```python
from build123d import *

# Parameters (mm, degrees)
SKETCH_1_R           = 11.65
SKETCH_1_R_2         = 1.8
EXTRUDE_1_DEPTH      = 170
SHELL_2_T            = -4
SKETCH_10_W          = 162
SKETCH_10_H          = 68.975267516
CUT_EXTRUDE_8_DEPTH  = 65
SKETCH_2_R           = 4
EXTRUDE_2_DEPTH      = 30
SKETCH_3_W           = 48.76473187
SKETCH_3_H           = 132
CUT_EXTRUDE_1_DEPTH  = 57
SKETCH_4_R           = 1.5
CUT_EXTRUDE_2_DEPTH  = 20
SKETCH_5_R           = 3.25
CUT_EXTRUDE_3_DEPTH  = 20
SKETCH_6_R           = 1.95
CUT_EXTRUDE_4_DEPTH  = 93
FILLET_1_R           = 4
CHAMFER_2_SIZE       = 6
SKETCH_7_W           = 70
SKETCH_7_H           = 15
CUT_EXTRUDE_5_DEPTH  = 39
SKETCH_9_W           = 25
SKETCH_9_H           = 25
CUT_EXTRUDE_7_DEPTH  = 39
SKETCH_11_R          = 1.75
CUT_EXTRUDE_9_DEPTH  = 10
SKETCH_8_W           = 19.8
SKETCH_8_H           = 13.4
CUT_EXTRUDE_10_DEPTH = 10
SKETCH_12_W          = 22
SKETCH_12_H          = 16
CUT_EXTRUDE_11_DEPTH = 1.2


with BuildPart() as part:
    # 草图1 → 凸台-拉伸1 (new body)
    with BuildSketch(Plane.XY):
        with BuildLine():
            Line((-6.571005291, -19.16114319), (73.428994709, -19.16114319))
            Line((73.428994709, -19.16114319), (73.428994709, 70.83885681))
            ThreePointArc((73.428994709, 70.83885681), (64.642198145, 92.052060245), (43.428994709, 100.83885681))
            Line((43.428994709, 100.83885681), (33.428994709, 100.83885681))
            Line((33.428994709, 100.83885681), (-46.571005291, 40.83885681))
            Line((-46.571005291, 40.83885681), (-46.571005291, 20.83885681))
            ThreePointArc((-46.571005291, 20.83885681), (-34.855276538, -7.445414438), (-6.571005291, -19.16114319))
        make_face()
        with Locations((3.428994709, 10.83885681)):
            Circle(SKETCH_1_R, mode=Mode.SUBTRACT)
        with Locations((43.428994709, 93.83885681)):
            Circle(SKETCH_1_R_2, mode=Mode.SUBTRACT)
        with Locations((65.87893903, 75.83885681)):
            Circle(SKETCH_1_R_2, mode=Mode.SUBTRACT)
    extrude(amount=EXTRUDE_1_DEPTH)

    # 抽壳2
    shell_2_openings = [part.faces().sort_by_distance(p)[0] for p in [
        (-6.571005291, 70.83885681, 85),
    ]]
    offset(amount=SHELL_2_T, openings=shell_2_openings)

    # 草图10 → 切除-拉伸8 (cut)
    with BuildSketch(Plane(origin=(73.428994709, 0, 0), x_dir=(0, 0, -1), z_dir=(1, 0, 0))):
        with Locations((-85, 95.326490568)):
            Rectangle(SKETCH_10_W, SKETCH_10_H)
    extrude(amount=-CUT_EXTRUDE_8_DEPTH, mode=Mode.SUBTRACT)

    # 草图2 → 凸台-拉伸2 (add)
    with BuildSketch(Plane(origin=(-36.368213173, 48.490950898, 0), x_dir=(0.8000000000000002, 0.6, 0), z_dir=(-0.6, 0.8000000000000002, 0))):
        with Locations((81.246509853, -6)):
            Circle(SKETCH_2_R)
        with Locations((-6.753490147, -6)):
            Circle(SKETCH_2_R)
        with Locations((81.246509853, -164)):
            Circle(SKETCH_2_R)
        with Locations((-6.753490147, -164)):
            Circle(SKETCH_2_R)
    extrude(amount=-EXTRUDE_2_DEPTH)

    # 草图3 → 切除-拉伸1 (cut)
    with BuildSketch(Plane(origin=(0, -12.16114319, 0), x_dir=(1, 0, 0), z_dir=(0, 1, 0))):
        with Locations((11.820994157, -85)):
            Rectangle(SKETCH_3_W, SKETCH_3_H)
    extrude(amount=CUT_EXTRUDE_1_DEPTH, mode=Mode.SUBTRACT)

    # 草图4 → 切除-拉伸2 (cut)
    with BuildSketch(Plane(origin=(-36.368213173, 48.490950898, 0), x_dir=(0.8000000000000002, 0.6, 0), z_dir=(-0.6, 0.8000000000000002, 0))):
        with Locations(Location((-6.753490147, -6, 0), (0, 0, 180))):
            Circle(SKETCH_4_R)
        with Locations((81.246509853, -6)):
            Circle(SKETCH_4_R)
        with Locations(Location((81.246509853, -164, 0), (0, 0, 180))):
            Circle(SKETCH_4_R)
        with Locations((-6.753490147, -164)):
            Circle(SKETCH_4_R)
    extrude(amount=-CUT_EXTRUDE_2_DEPTH, mode=Mode.SUBTRACT)

    # 草图5 → 切除-拉伸3 (cut)
    with BuildSketch(Plane(origin=(0, -15.16114319, 0), x_dir=(1, 0, 0), z_dir=(0, 1, 0))):
        with Locations(Location((23.428994709, -45, 0), (0, 0, 270))):
            Circle(SKETCH_5_R)
        with Locations(Location((39.428994709, -45, 0), (0, 0, 270))):
            Circle(SKETCH_5_R)
        with Locations(Location((23.428994709, -125, 0), (0, 0, 270))):
            Circle(SKETCH_5_R)
        with Locations(Location((39.428994709, -125, 0), (0, 0, 270))):
            Circle(SKETCH_5_R)
    extrude(amount=-CUT_EXTRUDE_3_DEPTH, mode=Mode.SUBTRACT)

    # 草图6 → 切除-拉伸4 (cut)
    with BuildSketch(Plane(origin=(0, 100.83885681, 0), x_dir=(1, 0, 0), z_dir=(0, 1, 0))):
        with Locations(Location((3.428994709, -158.5, 0), (0, 0, 270))):
            Circle(SKETCH_6_R)
        with Locations(Location((3.428994709, -11.5, 0), (0, 0, 270))):
            Circle(SKETCH_6_R)
    extrude(amount=-CUT_EXTRUDE_4_DEPTH, mode=Mode.SUBTRACT)

    # 圆角1
    fillet_1_edges = [part.edges().sort_by_distance(p)[0] for p in [
        (-12.221005291, 10.83885681, 4),
        (-12.221005291, 10.83885681, 166),
    ]]
    fillet(fillet_1_edges, radius=FILLET_1_R)

    # Chamfer 2
    chamfer_2_edges = [part.edges().sort_by_distance(p)[0] for p in [
        (-23.771005291, 20.43885681, 4),
        (46.628994709, 73.23885681, 4),
        (46.628994709, 73.23885681, 166),
        (-23.771005291, 20.43885681, 166),
    ]]
    chamfer(chamfer_2_edges, length=CHAMFER_2_SIZE - 0.0001)  # a hair under: the kernel refuses the full size

    # 草图7 → 切除-拉伸5 (cut)
    with BuildSketch(Plane(origin=(73.428994709, 0, 0), x_dir=(0, 0, -1), z_dir=(1, 0, 0))):
        with Locations((-85, 53.33885681)):
            Rectangle(SKETCH_7_W, SKETCH_7_H)
    extrude(amount=-CUT_EXTRUDE_5_DEPTH, mode=Mode.SUBTRACT)

    # 草图9 → 切除-拉伸7 (cut)
    with BuildSketch(Plane.XZ.offset(19.16114319)):
        with Locations((56.928994709, 153.5)):
            Rectangle(SKETCH_9_W, SKETCH_9_H)
    extrude(amount=-CUT_EXTRUDE_7_DEPTH, mode=Mode.SUBTRACT)

    # 草图11 → 切除-拉伸9 (cut)
    with BuildSketch(Plane.ZY.offset(-69.428994709)):
        with Locations((44.5, 51.83885681)):
            Circle(SKETCH_11_R)
        with Locations((44.5, 15.83885681)):
            Circle(SKETCH_11_R)
        with Locations((125.5, 15.83885681)):
            Circle(SKETCH_11_R)
        with Locations((125.5, 51.83885681)):
            Circle(SKETCH_11_R)
    extrude(amount=-CUT_EXTRUDE_9_DEPTH, mode=Mode.SUBTRACT)

    # 草图8 → 切除-拉伸10 (cut)
    with BuildSketch(Plane.XY.offset(170)):
        with Locations((33.528994709, 42.53885681)):
            Rectangle(SKETCH_8_W, SKETCH_8_H)
    extrude(amount=-CUT_EXTRUDE_10_DEPTH, mode=Mode.SUBTRACT)

    # 草图12 → 切除-拉伸11 (cut)
    with BuildSketch(Plane.XY.offset(170)):
        with Locations((33.528994709, 42.53885681)):
            Rectangle(SKETCH_12_W, SKETCH_12_H)
    extrude(amount=-CUT_EXTRUDE_11_DEPTH, mode=Mode.SUBTRACT)


solid = part.part
```
Geometry check sheet. Reference: the model listing, model coordinates, mm. A direction names the side the tool comes from. Round coordinates to 2 decimals unless told otherwise and drop trailing zeros. Order: outer loops, then holes, each group sorted by start corner. A loop starts at its lowest first (then second) coordinate and runs counter-clockwise, first axis right, second up. Notation, with made-up numbers: (59, 50.25) -> (65, 50.25) arc R33 ccw to (65, 80.25) -> close; hole circle Ø3 at (12, 50.5). An arc over 180 degrees is marked (long way). Return JSON: item names as keys, results as strings. Group by question number.
Q1. Release check for a two-part mould opening along X. For faces 4 (the flat face through (-45.276, 41.81, 84.603)), 5 (the flat face through (44.429, -17, 153)), 6 (the flat face through (71, 60.839, 143)) record: released by +X, released by -X, zero draft, split by the parting line, or undercut.
Q2. Section check B-B, the plane y = -11.5. Record the boundary of the cut face in (x, z).
Q3. Material ranges on probe 1 along Y at (x, z) = (72.2, 125.5); probe 2 along Z at (x, y) = (36.5, 79); probe 3 along Z at (x, y) = (-2, 23), recorded low to high. Write a range as from..to.
Q4. Section check C-C, the plane x = 61. Record the boundary of the cut face in (y, z).
Q5. Tool access check on faces 1 (the flat face through (26, 28, 0)), 2 (the cylindrical face through (0.04, -4.44, 156.42)), 3 (the flat face through (69.429, 20, 84)). Record the directions out of +Z, -Z, +X, -X, +Y, -Y that give a thin tool (end or side, any length) a straight path to the whole face; none if there is none.
Q6. Section check D-D, the plane x = -35.5. Count the separate pieces of the cut face and the enclosed holes in it, plus the area to 3 significant figures.
Q7. Gauge pin test, flat ends, axial feed: pin 1 (6 mm diameter, centred on x = 3, y = 16.5, fed in from -Z); pin 2 (1.4 mm diameter, centred on x = 31, z = 167, fed in from +Y); pin 3 (1 mm diameter, centred on x = 57.5, z = 49.5, fed in from +Y); pin 4 (1.2 mm diameter, centred on x = 72, z = 75.5, fed in from +Y). Record the tip position at first contact, or that the pin passes through.
Q8. Section check A-A, the plane z = 34. Record the boundary of the cut face in (x, y), plus the area to 3 significant figures.
Numbers:
{
 "1": {"face 4": "released by -X", "face 5": "undercut", "face 6": "zero draft"},
 "2": {"outline": "(-30.11, 0) -> (73.43, 0) -> (73.43, 170) -> (-30.11, 170) -> close; hole (-22.39, 4) -> (69.43, 4) -> (69.43, 166) -> (-22.39, 166) -> close"},
 "3": {"probe 1": "-19.16..14.09, 17.59..50.09, 53.59..60.84", "probe 2": "0..4, 166..170", "probe 3": "0..19, 151..170"},
 "4": {"outline": "(-19.16, 0) -> (95.15, 0) -> (95.15, 4) -> (-15.16, 4) -> (-15.16, 141) -> (-19.16, 141) -> close; (-19.16, 166) -> (95.15, 166) -> (95.15, 170) -> (-19.16, 170) -> close"},
 "5": {"face 1": "-Z, +X, -X, +Y, -Y", "face 2": "none", "face 3": "+Y"},
 "6": {"separate pieces": "1", "enclosed holes": "2", "area": "1,560 mm^2"},
 "7": {"pin 1": "through", "pin 2": "y = 99.54", "pin 3": "y = -15.16", "pin 4": "y = 45.84"},
 "8": {"outline": "(-46.57, 20.84) arc R40 ccw to (-6.57, -19.16) -> (73.43, -19.16) -> (73.43, 60.84) -> (69.43, 60.84) -> (69.43, -15.16) -> (-6.57, -15.16) arc R36 cw to (-42.57, 20.84) -> (-42.57, 43.84) -> (-46.57, 40.84) -> close", "area": "949 mm^2"}
}
